Verification items for the finished model (mm, model axes). Face numbers are marked on the shaded views. Round coordinates to 2 decimals unless told otherwise and drop trailing zeros. Loops run counter-clockwise (first coordinate to the right, second up) from the corner with the lowest first, then second, coordinate; pieces in that order, holes last.
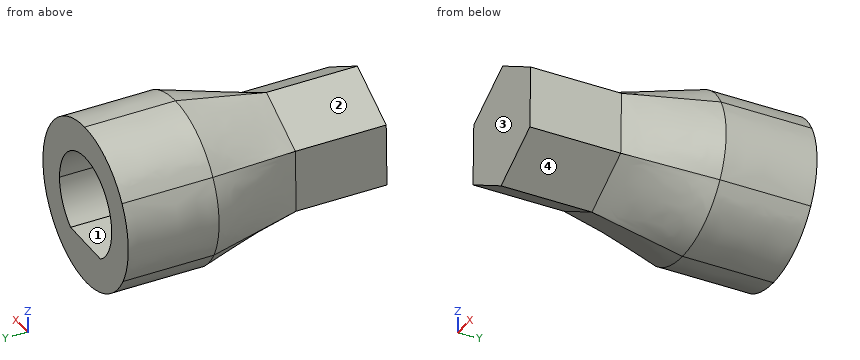
from build123d import *

# Parameters (mm, degrees)
F4_DEPTH = 5
F5_DEPTH = 5
F7_DEPTH = 5


# Not quite as in the source:
# - the arcs of a loft's sections are written as splines that run evenly, so that the points pair up as in the source's solid


with BuildPart() as f3:
    # F0 (on Front) → F3 section 0
    with BuildSketch(Plane.XZ):
        with BuildLine():
            add(Edge.make_bspline(
                [(3.8418426736, -2.3431271565), (4.1144778981, -1.8961084632), (4.3082439854, -1.4011386227), (4.5148518075, -0.3745248107), (4.5276427142, 0.1568666009), (4.3706679569, 1.1922320614), (4.2009409107, 1.6959513974), (3.9501289786, 2.1555697744)],
                knots=[0, 0, 0, 0, 0.3333333333, 0.3333333333, 0.6666666667, 0.6666666667, 1, 1, 1, 1], degree=3))
            add(Edge.make_bspline(
                [(3.9501289786, 2.1555697744), (3.6993170465, 2.6151881514), (3.3675436342, 3.0304794257), (2.5817739042, 3.7227139543), (2.1279708957, 3.9994869102), (1.1528307261, 4.3812255129), (0.6317334617, 4.4860972472), (0.1082863051, 4.4986969309)],
                knots=[0, 0, 0, 0, 0.3333333333, 0.3333333333, 0.6666666667, 0.6666666667, 1, 1, 1, 1], degree=3))
            add(Edge.make_bspline(
                [(0.1082863051, 4.4986969309), (-0.4151608516, 4.5112966146), (-0.9407003512, 4.4316180484), (-1.9330779034, 4.097238765), (-2.3996718185, 3.8426203093), (-3.2178372309, 3.1889934515), (-3.5692074491, 2.7901458498), (-3.8418426736, 2.3431271565)],
                knots=[0, 0, 0, 0, 0.3333333333, 0.3333333333, 0.6666666667, 0.6666666667, 1, 1, 1, 1], degree=3))
            add(Edge.make_bspline(
                [(-3.8418426736, 2.3431271565), (-4.1144778981, 1.8961084632), (-4.3082439854, 1.4011386227), (-4.5148518075, 0.3745248107), (-4.5276427142, -0.1568666009), (-4.3706679569, -1.1922320614), (-4.2009409107, -1.6959513974), (-3.9501289786, -2.1555697744)],
                knots=[0, 0, 0, 0, 0.3333333333, 0.3333333333, 0.6666666667, 0.6666666667, 1, 1, 1, 1], degree=3))
            add(Edge.make_bspline(
                [(-3.9501289786, -2.1555697744), (-3.6993170465, -2.6151881514), (-3.3675436342, -3.0304794257), (-2.5817739042, -3.7227139543), (-2.1279708957, -3.9994869102), (-1.1528307261, -4.3812255129), (-0.6317334617, -4.4860972472), (-0.1082863051, -4.4986969309)],
                knots=[0, 0, 0, 0, 0.3333333333, 0.3333333333, 0.6666666667, 0.6666666667, 1, 1, 1, 1], degree=3))
            add(Edge.make_bspline(
                [(-0.1082863051, -4.4986969309), (0.4151608516, -4.5112966146), (0.9407003512, -4.4316180484), (1.9330779034, -4.097238765), (2.3996718185, -3.8426203093), (3.2178372309, -3.1889934515), (3.5692074491, -2.7901458498), (3.8418426736, -2.3431271565)],
                knots=[0, 0, 0, 0, 0.3333333333, 0.3333333333, 0.6666666667, 0.6666666667, 1, 1, 1, 1], degree=3))
        make_face()
    # F2 (on offset) → F3 section 1
    with BuildSketch(Plane.XZ.offset(5)):
        Polygon((2.957451869, -1.8037401261), (3.0408107055, 1.659358386), (0.0833588365, 3.4630985121), (-2.957451869, 1.8037401261), (-3.0408107055, -1.659358386), (-0.0833588365, -3.4630985121), align=None)
    loft(ruled=True)

    # F4 (add): a face of the model
    f4_faces = [f3.faces().sort_by_distance(p)[0] for p in [
        (0, 0, 0),
    ]]
    extrude(f4_faces, amount=F4_DEPTH)

    # F5 (add): a face of the model
    f5_faces = [f3.faces().sort_by_distance(p)[0] for p in [
        (0, -5, 0),
    ]]
    extrude(f5_faces, amount=F5_DEPTH)

    # F6 (on Front) → F7 (cut)
    with BuildSketch(Plane.XZ):
        with BuildLine():
            ThreePointArc((1.5811388301, -2.25), (2.4403515918, -1.2677476518), (2.75, 0))
            ThreePointArc((2.75, 0), (-1.2677476518, 2.4403515918), (-1.5811388301, -2.25))
            Line((-1.5811388301, -2.25), (1.5811388301, -2.25))
        make_face()
    extrude(amount=-F7_DEPTH, mode=Mode.SUBTRACT)


solid = f3.part
1. Scan lines: L1, parallel to Z at x = 0, y = 2.65; L2, parallel to X at y = 1.6, z = 0; L3, parallel to Z at x = -1, y = 0.25. Record each from-to range of solid material in increasing order.
2. Section check A-A (y = -7). Enter the section's corners in (x, z), then the cut area to 3 significant figures.
3. Gauge pin test, flat ends, axial feed: P1, Ø1, axis at x = 3.5, y = 0, coming from the +Z side; P2, Ø1.5, axis at y = 0.5, z = 2.5, coming from the +X side. Record the tip position at first contact, or that the pin passes through.
4. Release check for a two-part mould opening along Z. For the marked faces 1, 2, 3 and 4 record: released by +Z, released by -Z, zero draft, split by the parting line, or undercut.
Taken from the geometry:
1. L1: z = -4.5 to -2.25, 2.75 to 4.5
1. L2: x = -4.5 to -2.75, 2.75 to 4.5
1. L3: z = -4.39 to -2.25, 2.56 to 4.39
2. outline: (-3.04, -1.66) - (-0.08, -3.46) - (2.96, -1.8) - (3.04, 1.66) - (0.08, 3.46) - (-2.96, 1.8) - close
2. area: 31.2 mm2
3. P1: stops at z = 3.35
3. P2: stops at x = 4.15
4. face 1: undercut
4. face 2: released by +Z
4. face 3: zero draft
4. face 4: released by -Z
